Read the model definition and answer for the solid it produces. Units are mm, in the model's axes. Face numbers are marked on the shaded views. Coordinates: 2 decimals unless noted, no trailing zeros. Loops run counter-clockwise (first coordinate to the right, second up) from the corner with the lowest first, then second, coordinate; pieces in that order, holes last.
Q1. Section A-A (z = 0) is taken. Give the vertices of the cut face in (x, y).
Q2. Straight lines are drawn through the part: line 1 (Y direction, x = 25.5, z = 0); line 2 (Y direction, x = 74.5, z = -1.5); line 3 (X direction, y = 12, z = 31). For each, find the intervals that lie inside material, in ascending order.
Q3. Section C-C (z = 27.5) is taken. Give the vertices of the cut face in (x, y), then the cut area to 3 significant figures.
Q4. Section D-D (y = 26) is taken. Give the vertices of the cut face in (x, z), then the cut area to 3 significant figures.
Q5. Flat-ended cylindrical pins translate along their axes: P1, Ø3, axis at x = 63.5, z = -14.5, coming from the -Y side; P2, Ø24, axis at y = 0, z = 0, coming from the +X side; P3, Ø10, axis at x = 58.5, z = 13.5, coming from the +Y side; P4, Ø1, axis at x = 33.5, z = -19, coming from the +Y side. Find the tip coordinate at first contact, or state that the pin passes through.
Q6. The mould has two halves that part along Y. Classify the marked faces 1, 2 and 3: pulls with the +Y half, pulls with the -Y half, needs draft (parallel to the pull), parting line crosses it, or undercut.
from build123d import *

# Parameters (mm, degrees)
FILLET1_R = 4


with BuildPart() as part:
    # Sketch1 → Revolve1 (revolve)
    with BuildSketch(Plane.XY, mode=Mode.PRIVATE) as revolve1_sk:
        Polygon((0, 20), (100, 20), (100, 30), (100, 35), (90, 35), (90, 30), (0, 30), align=None)
    revolve(revolve1_sk.sketch.rotate(Axis((0, 0, 0), (1, 0, 0)), 90), axis=Axis((0, 0, 0), (1, 0, 0)))

    # Fillet1
    fillet1_edges = [part.edges().sort_by_distance(p)[0] for p in [
        (0, 0, -20),
    ]]
    fillet(fillet1_edges, radius=FILLET1_R)


solid = part.part
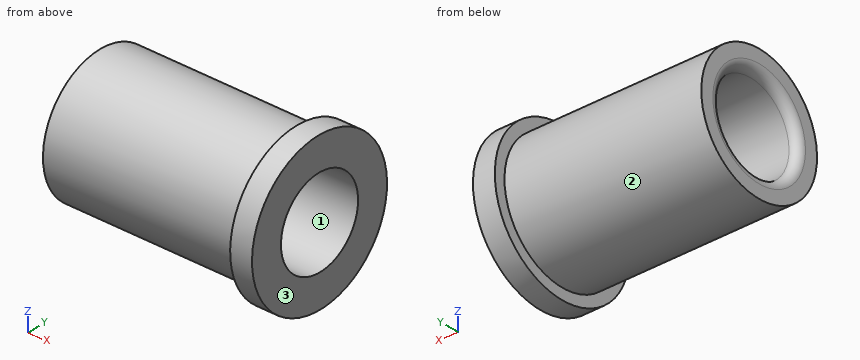
Numbers:
1. outline: (0, -30) - (90, -30) - (90, -35) - (100, -35) - (100, -20) - (4, -20) arc R4 ccw to (0, -24) - close; (0, 24) arc R4 ccw to (4, 20) - (100, 20) - (100, 35) - (90, 35) - (90, 30) - (0, 30) - close
2. line 1: y = -30 to -20, 20 to 30
2. line 2: y = -29.96 to -19.94, 19.94 to 29.96
2. line 3: x = 90 to 100
3. outline: (0, -11.99) - (90, -11.99) - (90, -21.65) - (100, -21.65) - (100, 21.65) - (90, 21.65) - (90, 11.99) - (0, 11.99) - close
3. area: 2,590 mm2
4. outline: (0, -14.97) - (90, -14.97) - (90, -23.43) - (100, -23.43) - (100, 23.43) - (90, 23.43) - (90, 14.97) - (0, 14.97) - close
4. area: 3,160 mm2
5. P1: stops at y = -27.04
5. P2: passes through
5. P3: stops at y = 28.77
5. P4: stops at y = 23.62
6. face 1: undercut
6. face 2: parting line crosses it
6. face 3: needs draft
